The listing builds one solid part. Answer for the finished solid, in the listing's coordinates (mm). A direction names the side the tool comes from. Give positions to 0.01 mm unless a question says otherwise; leave off trailing zeros. Write each loop counter-clockwise with the first axis right and the second up, starting at its lowest first coordinate (ties: lowest second). Pieces come first, ordered by that corner, then holes. Notation, with made-up numbers: (22, -30) - (72, -30) arc R14 ccw to (72, -11) - close; hole circle Ø1 at (71, 86.5). An arc over 180 degrees is marked (long way). Use a Markdown table: item, result. Add a question column.
from build123d import *

# Parameters (mm, degrees)
SKETCH1_W                = 29
SKETCH1_H                = 15.3
BOSS_EXTRUDE1_DEPTH      = 1.3
BOSS_EXTRUDE2_DEPTH      = 4.1
SKETCH3_W                = 0.65
SKETCH3_H                = 0.65
BOSS_EXTRUDE3_DEPTH      = 1.4
BOSS_EXTRUDE3_DEPTH_BACK = 10
SKETCH4_W                = 4.99
SKETCH4_H                = 10.07
BOSS_EXTRUDE4_DEPTH      = 2.54
SKETCH5_W                = 4
SKETCH5_H                = 4
BOSS_EXTRUDE5_DEPTH      = 0.65
FILLET1_R                = 0.25
CHAMFER1_SIZE            = 0.15
BOSS_EXTRUDE6_DEPTH      = 0.1


with BuildPart() as part:
    # Sketch1 → Boss-Extrude1 (new body)
    with BuildSketch(Plane(origin=(0, 0, 0), x_dir=(1, 0, 0), z_dir=(0, 1, 0))):
        with Locations((-0.556382979, -0.474734043)):
            Rectangle(SKETCH1_W, SKETCH1_H)
    extrude(amount=BOSS_EXTRUDE1_DEPTH)

    # Sketch2 → Boss-Extrude2 (add)
    with BuildSketch(Plane(origin=(0, 1.3, 0), x_dir=(1, 0, 0), z_dir=(0, 1, 0))):
        with BuildLine():
            Line((-6.806382979, -4.574734043), (-0.256382979, -4.574734043))
            ThreePointArc((-0.256382979, -4.574734043), (1.493617021, -6.324734043), (-0.256382979, -8.074734043))
            Line((-0.256382979, -8.074734043), (-6.806382979, -8.074734043))
            ThreePointArc((-6.806382979, -8.074734043), (-8.556382979, -6.324734043), (-6.806382979, -4.574734043))
        make_face()
    extrude(amount=BOSS_EXTRUDE2_DEPTH)

    # Sketch3 → Boss-Extrude3 (add, two sides)
    with BuildSketch(Plane(origin=(0, 1.3, 0), x_dir=(1, 0, 0), z_dir=(0, 1, 0))) as boss_extrude3_sk:
        with Locations((-13.131382979, 4.950265957)):
            Rectangle(SKETCH3_W, SKETCH3_H)
        with Locations((-10.591382979, 4.950265957)):
            Rectangle(SKETCH3_W, SKETCH3_H)
        with Locations((-10.591382979, 2.410265957)):
            Rectangle(SKETCH3_W, SKETCH3_H)
        with Locations((-10.591382979, -0.129734043)):
            Rectangle(SKETCH3_W, SKETCH3_H)
        with Locations((-10.591382979, -2.669734043)):
            Rectangle(SKETCH3_W, SKETCH3_H)
        with Locations((-13.131382979, 2.410265957)):
            Rectangle(SKETCH3_W, SKETCH3_H)
        with Locations((-13.131382979, -0.129734043)):
            Rectangle(SKETCH3_W, SKETCH3_H)
        with Locations((-13.131382979, -2.669734043)):
            Rectangle(SKETCH3_W, SKETCH3_H)
    extrude(amount=BOSS_EXTRUDE3_DEPTH)
    extrude(boss_extrude3_sk.sketch, amount=-BOSS_EXTRUDE3_DEPTH_BACK)

    # Sketch4 → Boss-Extrude4 (add)
    with BuildSketch(Plane.XZ):
        with Locations((-11.861382979, -1.140265957)):
            Rectangle(SKETCH4_W, SKETCH4_H)
    extrude(amount=BOSS_EXTRUDE4_DEPTH)

    # Sketch5 → Boss-Extrude5 (add)
    with BuildSketch(Plane(origin=(0, 1.3, 0), x_dir=(1, 0, 0), z_dir=(0, 1, 0))):
        with Locations((-3.406382979, 0.875265957)):
            Rectangle(SKETCH5_W, SKETCH5_H)
    extrude(amount=BOSS_EXTRUDE5_DEPTH)

    # Fillet1
    fillet1_edges = [part.edges().sort_by_distance(p)[0] for p in [
        (-8.556382979, 5.4, 6.324734043),
        (-3.531382979, 5.4, 8.074734043),
        (1.493617021, 5.4, 6.324734043),
        (-3.531382979, 5.4, 4.574734043),
    ]]
    fillet(fillet1_edges, radius=FILLET1_R)

    # Chamfer1
    chamfer1_edges = [part.edges().sort_by_distance(p)[0] for p in [
        (-10.591382979, -8.7, 2.344734043),
        (-10.266382979, -8.7, 2.669734043),
        (-10.591382979, -8.7, 2.994734043),
        (-10.916382979, -8.7, 2.669734043),
        (-13.131382979, -8.7, -2.735265957),
        (-12.806382979, -8.7, -2.410265957),
        (-13.131382979, -8.7, -2.085265957),
        (-13.456382979, -8.7, -2.410265957),
        (-13.131382979, -8.7, -0.195265957),
        (-12.806382979, -8.7, 0.129734043),
        (-13.131382979, -8.7, 0.454734043),
        (-13.456382979, -8.7, 0.129734043),
        (-13.131382979, -8.7, 2.344734043),
        (-12.806382979, -8.7, 2.669734043),
        (-13.131382979, -8.7, 2.994734043),
        (-13.456382979, -8.7, 2.669734043),
        (-13.456382979, -8.7, -4.950265957),
        (-13.131382979, -8.7, -5.275265957),
        (-12.806382979, -8.7, -4.950265957),
        (-13.131382979, -8.7, -4.625265957),
        (-10.591382979, -8.7, -5.275265957),
        (-10.266382979, -8.7, -4.950265957),
        (-10.591382979, -8.7, -4.625265957),
        (-10.916382979, -8.7, -4.950265957),
        (-10.591382979, -8.7, -2.735265957),
        (-10.266382979, -8.7, -2.410265957),
        (-10.591382979, -8.7, -2.085265957),
        (-10.916382979, -8.7, -2.410265957),
        (-10.591382979, -8.7, -0.195265957),
        (-10.266382979, -8.7, 0.129734043),
        (-10.591382979, -8.7, 0.454734043),
        (-10.916382979, -8.7, 0.129734043),
    ]]
    chamfer(chamfer1_edges, length=CHAMFER1_SIZE)

    # Sketch6 → Boss-Extrude6 (add)
    with BuildSketch(Plane(origin=(0, 1.3, 0), x_dir=(1, 0, 0), z_dir=(0, 1, 0))):
        Polygon((4.693617021, 4.173262585), (13.693617021, 4.173262585), (13.693617021, 2.373262585), (9.693617021, 2.373262585), (9.693617021, 1.573262585), (13.693617021, 1.573262585), (13.693617021, -0.226737415), (9.693617021, -0.226737415), (9.693617021, -1.026737415), (13.693617021, -1.026737415), (13.693617021, -2.826737415), (9.693617021, -2.826737415), (9.693617021, -3.626737415), (13.693617021, -3.626737415), (13.693617021, -7.962396389), (13.193617021, -7.962396389), (13.193617021, -4.126737415), (9.193617021, -4.126737415), (9.193617021, -2.326737415), (13.193617021, -2.326737415), (13.193617021, -1.526737415), (9.193617021, -1.526737415), (9.193617021, 0.273262585), (13.193617021, 0.273262585), (13.193617021, 1.073262585), (9.193617021, 1.073262585), (9.193617021, 2.873262585), (13.193617021, 2.873262585), (13.193617021, 3.673262585), (7.693617021, 3.673262585), (7.693617021, -4.126737415), (7.193617021, -4.126737415), (7.193617021, 3.671905646), (4.693617021, 3.671905646), align=None)
    extrude(amount=BOSS_EXTRUDE6_DEPTH)


solid = part.part
1. The part is cut by section A-A (y = -5.25). Count the separate pieces of the cut face and the enclosed holes in it, and give its area (3 significant figures).
2. Given P1, Ø2, axis at y = -1.5, z = 0, coming from the +X side; P2, Ø1.2, axis at x = -2.5, y = 3.5, coming from the -Z side; P3, Ø5, axis at y = 4, z = 6.5, coming from the -X side, each flat-ended and moving along its own axis, determine where each tip first touches the part or whether it passes through.
3. The part is cut by section B-B (x = -3.75). Give the vertices of the cut face in (y, z), and give its area (3 significant figures).
4. Which of the six approach directions +Z, -Z, +X, -X, +Y, -Y give full straight-line access (tool end or side, diameter ignored) to faces 1 (the flat face through (11, 1.4, 0)), 2 (the flat face through (-9.366, -1, -1)), 3 (the flat face through (-14.356, -1, -1)), 4 (the flat face through (-3, 3, 8.075)), 5 (the flat face through (-12, -1, -6.175))?
5. Consider L1, parallel to X at y = -6, z = -4.75; L2, parallel to Z at x = -3.75, y = 1.5; L3, parallel to Y at x = -7, z = 1. Determine where each line is inside the solid, lowest interval first. Write a range as [from, to].
6. The part is cut by section D-D (x = 3). Give the vertices of the cut face in (y, z).
7. The part is cut by section C-C (y = -1.75). Give the vertices of the cut face in (x, z).
Check values:
| question | item | result |
|---|---|---|
| 1 | separate pieces | 8 |
| 1 | enclosed holes | 0 |
| 1 | area | 3.38 mm2 |
| 2 | P1 | stops at x = -9.37 |
| 2 | P2 | stops at z = 4.57 |
| 2 | P3 | stops at x = -8.56 |
| 3 | outline | (0, -7.18) - (1.3, -7.18) - (1.3, -2.88) - (1.95, -2.88) - (1.95, 1.12) - (1.3, 1.12) - (1.3, 4.57) - (5.15, 4.57) arc R0.25 ccw to (5.4, 4.82) - (5.4, 7.82) arc R0.25 ccw to (5.15, 8.07) - (1.3, 8.07) - (1.3, 8.12) - (0, 8.12) - close |
| 3 | area | 36.8 mm2 |
| 4 | face 1 | +Z, -Z, +X, +Y |
| 4 | face 2 | +Z, -Z, +X, -Y |
| 4 | face 3 | +Z, -Z, -X, -Y |
| 4 | face 4 | +Z, +X, -X, +Y |
| 4 | face 5 | -Z, +X, -X, -Y |
| 5 | L1 | x = [-13.46, -12.81], [-10.92, -10.27] |
| 5 | L2 | z = [-2.88, 1.12], [4.57, 8.07] |
| 5 | L3 | y = [0, 1.3] |
| 6 | outline | (0, -7.18) - (1.3, -7.18) - (1.3, 8.12) - (0, 8.12) - close |
| 7 | outline | (-14.36, -6.18) - (-9.37, -6.18) - (-9.37, 3.89) - (-14.36, 3.89) - close |
